Could you check a few things on this drawing? It's one solid part, dimensions in mm from its lowest x, y, z. Coordinates: 2 decimals unless noted, no trailing zeros. Write each loop counter-clockwise with the first axis right and the second up, starting at its lowest first coordinate (ties: lowest second). Pieces come first, ordered by that corner, then holes.
Item 1: I want a section at D-D (y = 232). Please give me the cut outline in (x, z) (3 decimals), and give its area (3 significant figures).
Item 2: Please list where these lines run through material, in increasing order: line 1 (Y direction, x = 69, z = 1.75); line 2 (Y direction, x = 59, z = 3.05); line 3 (Y direction, x = 130.5, z = 1.1).
Item 3: I want a section at C-C (z = 0.9). Please give me the cut outline in (x, y) (3 decimals).
Item 4: I want a section at A-A (x = 23.5). Please give me the cut outline in (y, z) (3 decimals).
Item 5: I want a section at B-B (x = 73). Please give me the cut outline in (y, z) (3 decimals), and give its area (3 significant figures).
Item 6: I'm going to push flat-ended pins straight in: P1, Ø1.5, axis at x = 94.5, z = 1, coming from the +Y side; P2, Ø1.6, axis at x = 102.5, z = 1.5, coming from the +Y side. Where does each tip first touch, or does it pass through?
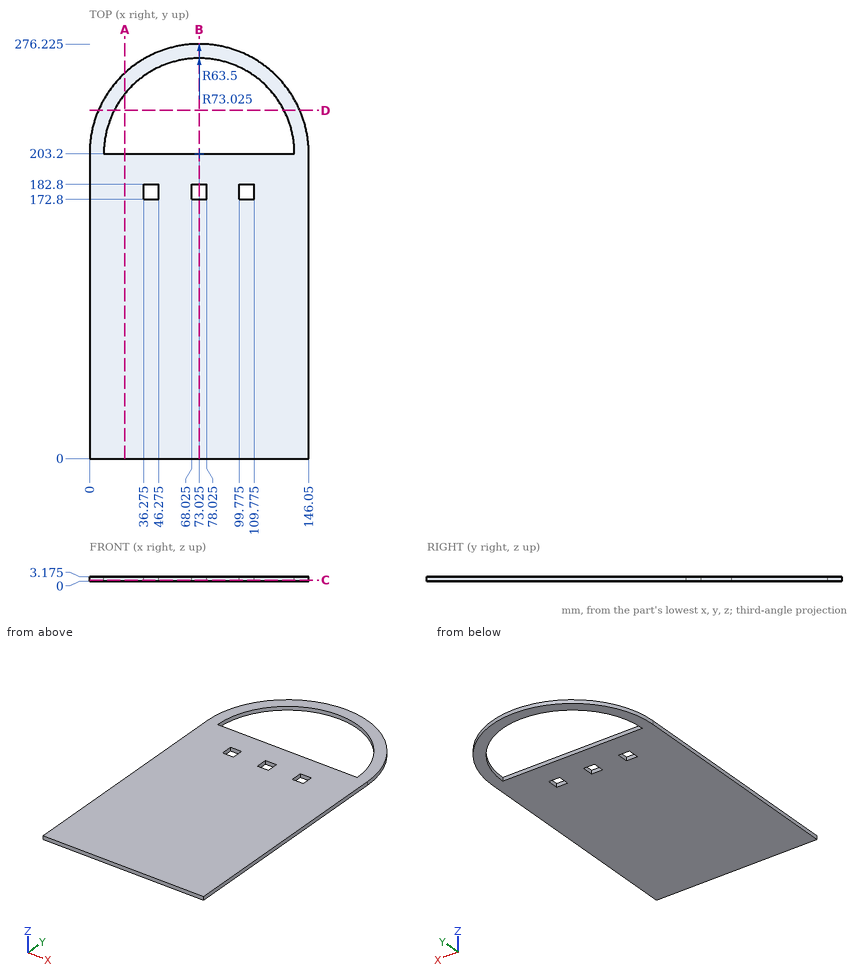
Answer:
1. outline: (5.919, 0) - (16.432, 0) - (16.432, 3.175) - (5.919, 3.175) - close; (129.618, 0) - (140.131, 0) - (140.131, 3.175) - (129.618, 3.175) - close
1. area: 66.8 mm2
2. line 1: y = 0 to 172.8, 182.8 to 203.2, 266.57 to 276.11
2. line 2: y = 0 to 203.2, 265.13 to 274.87
2. line 3: y = 0 to 203.2, 230.2 to 248.25
3. outline: (0, 0) - (146.05, 0) - (146.05, 203.2) arc R73.025 ccw to (0, 203.2) - close; hole (9.525, 203.2) - (136.525, 203.2) arc R63.5 ccw to start; hole (36.275, 172.8) - (46.275, 172.8) - (46.275, 182.8) - (36.275, 182.8) - close; hole (68.025, 172.8) - (78.025, 172.8) - (78.025, 182.8) - (68.025, 182.8) - close; hole (99.775, 172.8) - (109.775, 172.8) - (109.775, 182.8) - (99.775, 182.8) - close
4. outline: (0, 0) - (203.2, 0) - (203.2, 3.175) - (0, 3.175) - close; (242.943, 0) - (256.865, 0) - (256.865, 3.175) - (242.943, 3.175) - close
5. outline: (0, 0) - (172.8, 0) - (172.8, 3.175) - (0, 3.175) - close; (182.8, 0) - (203.2, 0) - (203.2, 3.175) - (182.8, 3.175) - close; (266.7, 0) - (276.225, 0) - (276.225, 3.175) - (266.7, 3.175) - close
5. area: 644 mm2
6. P1: stops at y = 273.22
6. P2: stops at y = 270.36
